Design review of the part built by this model. Coordinates are the model's own, in mm. A direction names the side the tool comes from. Coordinates: 2 decimals unless noted, no trailing zeros. Write each loop counter-clockwise with the first axis right and the second up, starting at its lowest first coordinate (ties: lowest second). Pieces come first, ordered by that corner, then holes.
Q1. Take a section at D-D, the plane y = 29. Write out the cut boundary in (x, z), plus the area to 3 significant figures.
Q2. Take a section at C-C, the plane z = 105. Write out the cut boundary in (x, y).
Q3. For L1, parallel to Y at x = -116, z = 143.5; L2, parallel to X at y = 29, z = 95; L3, parallel to Y at x = 0, z = 92.25, list the stretches that pass through material, from the lowest coordinate up.
Q4. The part is to be moulded in two halves that separate along X. For faces 1 (the cylindrical face through (-28.289, -68.196, 118.699)), 2 (the cylindrical face through (-0.705, 32.173, 93.251)), 3 (the flat face through (-3, -70, 121)), 4 (the cylindrical face through (3.461, 53.972, 96.454)), say which applies: released by +X, released by -X, zero draft, split by the parting line, or undercut.
Q5. Take a section at A-A, the plane y = -55. Write out the cut boundary in (x, z), plus the area to 3 significant figures.
Q6. Take a section at B-B, the plane x = -101. Write out the cut boundary in (y, z).
Q7. For faces 5 (the flat face through (-74, 31, 117)), 6 (the flat face through (-74, 37, 145.3)), 7 (the flat face through (-3, 52, 152)), 8 (the flat face through (0, 29, 96.8)), list the 3-axis set-ups (+Z, -Z, +X, -X, +Y, -Y) from which the entire face can be reached by the end or side of a thin tool; tool diameter is ignored.
Q8. For pin 1 Ø3.5 at (x, y) = (-79, 37) entering from +Z; pin 2 Ø6 at (x, z) = (-54.5, 102.5) entering from -Y; pin 3 Ø3 at (x, z) = (-45, 128) entering from +Y, all flat-tipped, find the tip position at first contact; note any pin that passes through.
from build123d import *

# Parameters (mm, degrees)
SKETCH068_W     = 55
SKETCH068_H     = 122
PAD033_DEPTH    = 63
SKETCH069_R     = 27.5
PAD034_DEPTH    = 4
SKETCH070_R     = 3.25
POCKET026_DEPTH = 7
SKETCH071_W     = 11
SKETCH071_H     = 55.5
PAD035_DEPTH    = 92
FILLET_R        = 6
FILLET001_R     = 2


with BuildPart() as part:
    # Sketch068 (on Face5 of ShapeBinder026) → Pad033 (new body)
    with BuildSketch(Plane.XY.offset(89.8)):
        with Locations((-2.5, -9)):
            Rectangle(SKETCH068_W, SKETCH068_H)
    extrude(amount=PAD033_DEPTH)

    # Sketch069 (on Face1 of Pad033) → Pad034 (join)
    with BuildSketch(Plane(origin=(0, 52, -4), x_dir=(-1, 0, 0), z_dir=(0, 1, 0))):
        with Locations((2.5, 127.3)):
            Circle(SKETCH069_R)
    extrude(amount=PAD034_DEPTH)

    # Sketch070 (on Face5 of Pad033) → Pocket026 (cut)
    with BuildSketch(Plane(origin=(0, 0, 89.8), x_dir=(1, 0, 0), z_dir=(0, 0, -1))):
        with Locations((0, -29)):
            Circle(SKETCH070_R)
    extrude(amount=-POCKET026_DEPTH, mode=Mode.SUBTRACT)

    # Sketch071 (on Face4 of Pad033) → Pad035 (join)
    with BuildSketch(Plane(origin=(-30, 0, -4), x_dir=(0, -1, 0), z_dir=(-1, 0, 0))):
        with Locations((-36.5, 121.55)):
            Rectangle(SKETCH071_W, SKETCH071_H)
    extrude(amount=PAD035_DEPTH)

    # Fillet
    fillet_edges = [part.edges().sort_by_distance(p)[0] for p in [
        (-30, -9, 152.8),
        (-30, -70, 121.3),
        (-2.5, -70, 89.8),
        (25, -9, 152.8),
        (-2.5, -70, 152.8),
        (25, -70, 121.3),
        (25, -9, 89.8),
    ]]
    fillet(fillet_edges, radius=FILLET_R)

    # Fillet001
    fillet001_edges = [part.edges().sort_by_distance(p)[0] for p in [
        (-76, 31, 145.3),
        (-122, 31, 117.55),
        (-76, 42, 145.3),
        (-122, 36.5, 145.3),
        (-122, 42, 117.55),
        (-122, 36.5, 89.8),
        (-76, 42, 89.8),
        (-76, 31, 89.8),
    ]]
    fillet(fillet001_edges, radius=FILLET001_R)


solid = part.part
Responses:
1. outline: (-30, 89.8) - (-3.25, 89.8) - (-3.25, 96.8) - (3.25, 96.8) - (3.25, 89.8) - (19, 89.8) arc R6 ccw to (25, 95.8) - (25, 146.8) arc R6 ccw to (19, 152.8) - (-24, 152.8) arc R6 ccw to (-30, 146.8) - close
1. area: 3,400 mm2
2. outline: (-122, 33) arc R2 ccw to (-120, 31) - (-30, 31) - (-30, -64) arc R6 ccw to (-24, -70) - (19, -70) arc R6 ccw to (25, -64) - (25, 52) - (18.03, 52) - (18.03, 56) - (-23.03, 56) - (-23.03, 52) - (-30, 52) - (-30, 42) - (-120, 42) arc R2 ccw to (-122, 40) - close
3. L1: y = 31.01 to 41.99
3. L2: x = -30 to -3.25, 3.25 to 24.95
3. L3: y = -68.84 to 25.75, 32.25 to 52
4. face 1: released by -X
4. face 2: undercut
4. face 3: zero draft
4. face 4: split by the parting line
5. outline: (-30, 89.8) - (19, 89.8) arc R6 ccw to (25, 95.8) - (25, 146.8) arc R6 ccw to (19, 152.8) - (-24, 152.8) arc R6 ccw to (-30, 146.8) - close
5. area: 3,440 mm2
6. outline: (31, 91.8) arc R2 ccw to (33, 89.8) - (40, 89.8) arc R2 ccw to (42, 91.8) - (42, 143.3) arc R2 ccw to (40, 145.3) - (33, 145.3) arc R2 ccw to (31, 143.3) - close
7. face 5: +Z, -Z, -X, -Y
7. face 6: +Z, -X, +Y, -Y
7. face 7: +Z, +Y
7. face 8: -Z
8. pin 1: stops at z = 145.3
8. pin 2: stops at y = 31
8. pin 3: stops at y = 42
